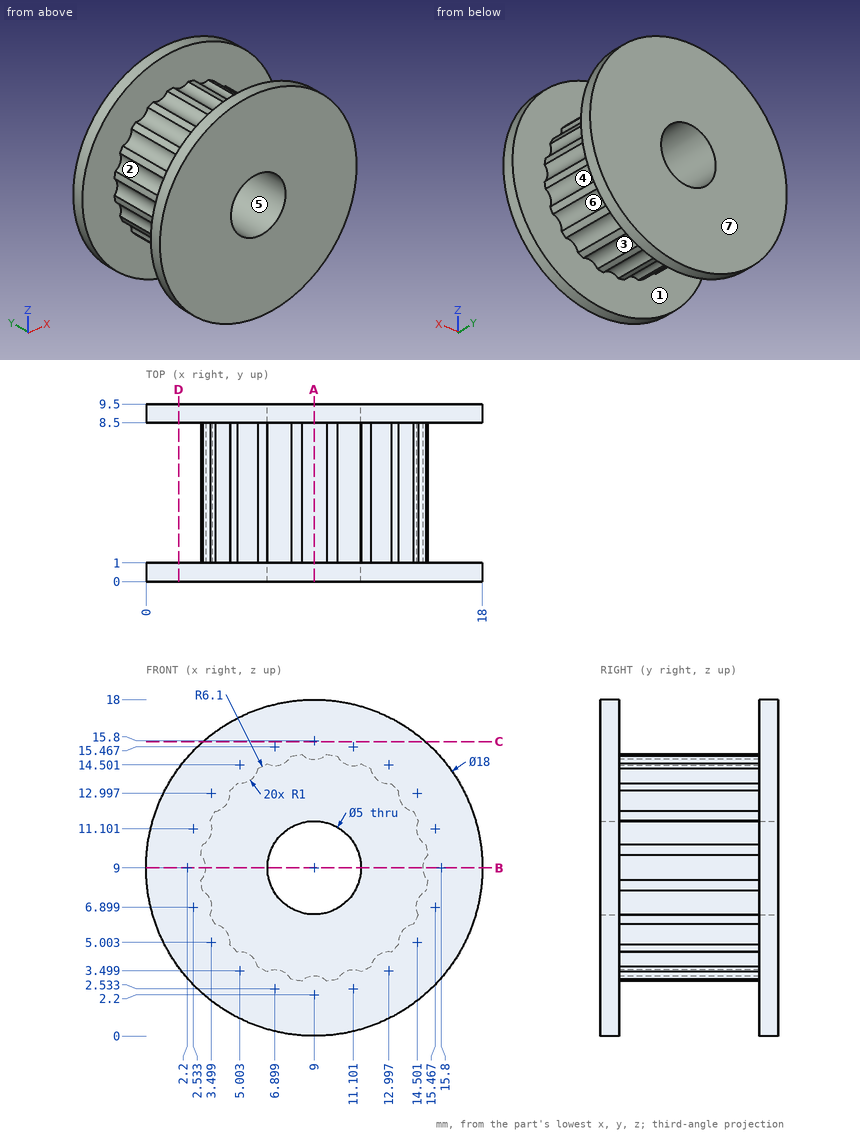
For this review, use the dimensioned drawing (mm, ordinates from the lowest corner) and the shaded views. A direction names the side the tool comes from. Give positions to 0.01 mm unless a question says otherwise; leave off trailing zeros. Write each loop counter-clockwise with the first axis right and the second up, starting at its lowest first coordinate (ties: lowest second). Pieces come first, ordered by that corner, then holes. Notation, with made-up numbers: M 24,-27 L 82,-27 A11 ccw 82,-23 Z; hole C -24,43.25 d6. An arc over 180 degrees is marked long. Answer as a JSON object with one key per item and string values. Group by question number.
1) We need section D-D (x = 1.75). Give the boundary of the cut face in (y, z).
2) For line 1 along Y through (x, z) = (16.5, 10.25); line 2 along X through (y, z) = (3.5, 9), list the stretches that pass through material, from the lowest coordinate up.
3) We need section B-B (z = 9). Give the boundary of the cut face in (x, y).
4) We need section A-A (x = 9). Give the boundary of the cut face in (y, z).
5) Clearance check with flat-ended pins moving along their axes: pin 1 Ø2 at (y, z) = (4.5, 8) entering from +X; pin 2 Ø1 at (x, y) = (14.5, 5.5) entering from +Z; pin 3 Ø3 at (x, y) = (15, 8) entering from +Z (1 decimal); pin 4 Ø6 at (x, z) = (9, 9) entering from -Y. State where each tip first meets the part, or that it passes through.
6) Mouldability with a two-part tool opening along Y and no side actions: class the marked faces 5, 6 and 7 as released by +Y, released by -Y, zero draft, split by the parting line, or undercut.
7) We need section C-C (z = 15.75). Give the boundary of the cut face in (x, y).
8) Tool access review of the marked faces 1, 2, 3 and 4: name each direction out of +Z, -Z, +X, -X, +Y, -Y from which nothing blocks a thin tool from reaching the whole face with its end or side.
Answer key:
{
 "1": {"outline": "M 0,3.67 L 1,3.67 L 1,14.33 L 0,14.33 Z; M 8.5,3.67 L 9.5,3.67 L 9.5,14.33 L 8.5,14.33 Z"},
 "2": {"line 1": "y = 0 to 1, 8.5 to 9.5", "line 2": "x = 3.2 to 6.5, 11.5 to 14.8"},
 "3": {"outline": "M 0,0 L 6.5,0 L 6.5,9.5 L 0,9.5 L 0,8.5 L 3.2,8.5 L 3.2,1 L 0,1 Z; M 11.5,0 L 18,0 L 18,1 L 14.8,1 L 14.8,8.5 L 18,8.5 L 18,9.5 L 11.5,9.5 Z"},
 "4": {"outline": "M 0,0 L 1,0 L 1,3.2 L 8.5,3.2 L 8.5,0 L 9.5,0 L 9.5,6.5 L 0,6.5 Z; M 0,11.5 L 9.5,11.5 L 9.5,18 L 8.5,18 L 8.5,14.8 L 1,14.8 L 1,18 L 0,18 Z"},
 "5": {"pin 1": "stops at x = 15.06", "pin 2": "stops at z = 12.13", "pin 3": "stops at z = 16.7", "pin 4": "stops at y = 0"},
 "6": {"face 5": "zero draft", "face 6": "undercut", "face 7": "released by +Y"},
 "7": {"outline": "M 3.05,0 L 14.95,0 L 14.95,1 L 3.05,1 Z; M 3.05,8.5 L 14.95,8.5 L 14.95,9.5 L 3.05,9.5 Z"},
 "8": {"face 1": "none", "face 2": "-X", "face 3": "-Z", "face 4": "+X"}
}
